Can you work these out from the model? Positions are in its coordinate system, mm. A direction names the side the tool comes from. Coordinates: 2 decimals unless noted, no trailing zeros. Order: outer loops, then holes, each group sorted by start corner. A loop starts at its lowest first (then second) coordinate and runs counter-clockwise, first axis right, second up. Notation, with made-up numbers: (36.25, 19.25) -> (56.25, 19.25) arc R10 cw to (56.25, 38.25) -> close; hole circle Ø10 at (-35.75, 37). An arc over 180 degrees is marked (long way). Return JSON: item names as keys, results as strings. Group by question number.
1) For pin 1 (3 mm diameter, centred on y = 23, z = -14.5, fed in from -X); pin 2 (14 mm diameter, centred on x = 27, z = 3.5, fed in from +Y); pin 3 (3 mm diameter, centred on x = 5.5, y = -11, fed in from -Z), each with a flat end and sliding along its axis, tell me the tip position at first contact or that it passes through.
2) For faces 5 (the flat face through (-34, 9, 18)), 6 (the flat face through (0, 0, 24)), 7 (the flat face through (1, 0, 22)), 8 (the cylindrical face through (45.186, 19.524, 7.336)), 9 (the flat face through (33, 25, 8)), which set-ups out of +Z, -Z, +X, -X, +Y, -Y let a thin tool reach every point of the face, with its end or its side?
3) Thinking about a two-plate mould opening in X: for faces 1 (the flat face through (-36.2, 9.1, 20)), 2 (the flat face through (33.4, 11.4, -18)), 3 (the cylindrical face through (-8.02, -36.12, -20.99)), 4 (the flat face through (46.2, -17, 14)), which applies, +X half, -X half, draft (parallel to the pull), parting line (faces both ways), or undercut?
4) If we section it at A-A, the plane y = 0: State how many separate pieces and enclosed holes the cut face has, then the cut area to 3 significant figures.
5) If we section it at C-C, the plane z = 3: Please give me the cut outline in (x, y), then the cut area to 3 significant figures.
6) If we section it at B-B, the plane x = -27: Please give me the cut outline in (y, z), then the cut area to 3 significant figures.
7) If I drill on probe 1 along Z at (x, y) = (33.5, 12); probe 2 along Z at (x, y) = (-19, -29.5); probe 3 along Y at (x, z) = (40, 6), over which ranges is the centre line in solid material (lowest first)? Write a range as from..to.
Autodesk Inventor part; units mm, degrees
ref_plane "作業平面1" through (0, 0, 0) normal (1, 0, 0) x (0, 1, 0)
ref_plane "YZ Plane" through (0, 0, 0) normal (1, 0, 0) x (0, 1, 0)
ref_plane "XZ Plane" through (0, 0, 0) normal (0, 1, 0) x (-1, 0, 0)
sketch "ｽｹｯﾁ1" plane through (0, 0, 0) normal (0, 0, 1) x (1, 0, 0)
  circle A0 centre (0, 0) radius 40
  dimension "d0" = 80
extrude "押し出し1" add sketch "ｽｹｯﾁ1" along normal mid plane 40
sketch "ｽｹｯﾁ2" plane through (0, 0, 20) normal (0, 0, 1) x (1, 0, 0)
  circle A0 centre (0, 0) radius 40
  circle A1 centre (0, 0) radius 37
  dimension "d3" = 3
extrude "押し出し2" add sketch "ｽｹｯﾁ2" along normal blind 2 contours A1
mirror "Mirror1" about plane through (0, 0, 0) normal (0, 0, 1) of "押し出し2"
ref_plane "作業平面1" through (0, 0, 0) normal (1, 0, 0) x (0, 1, 0)
sketch "ｽｹｯﾁ3" plane through (0, 0, 0) normal (1, 0, 0) x (0, 1, 0)
  line L0 (-37, -22) -> (37, -22)
  line L1 (40, -20) -> (-40, -20)
  line L2 (-25, 26) -> (25, 26)
  line L3 (25, 26) -> (25, -20)
  line L4 (25, -20) -> (-25, -20)
  line L5 (-25, -20) -> (-25, 26)
  line L6 (-25, 3) -> (25, 3)
  line L7 (0, 26) -> (0, -20)
  line L8 (0, -20) -> (0, 24.715)
  dimension "d6" = 50
  dimension "d7" = 46
  dimension "d8" = 25
extrude "押し出し3" add sketch "ｽｹｯﾁ3" along normal blind 46.2
sketch "Sketch4" plane through (46.2, 0, 0) normal (1, 0, 0) x (0, 0, -1)
  point P0 (0, 0)
ref_plane "Work Plane2" through (46.2, 0, -20) normal (0, -1, 0) x (1, 0, 0)
ref_plane "Work Plane3" through (46.2, 25, 3) normal (0, 0, -1) x (-1, 0, 0)
shell "Shell1" thickness 2 removed faces 0
sketch "Sketch7" plane through (0, 0, 22) normal (0, 0, 1) x (1, 0, 0)
  circle A0 centre (0, 0) radius 37
hole "Hole1" at (0, 0, 22) direction (0, 0, -1) diameter 50 end through all
sketch "Sketch8" plane through (46.2, 0, 0) normal (1, 0, 0) x (0, 0, -1)
  point P0 (-3, 0)
hole "Hole2" at (46.2, 0, 3) direction (-1, 0, 0) diameter 40 depth 2 tip angle 118
sketch "Sketch9" plane through (0, 0, -22) normal (0, 0, -1) x (-1, 0, 0)
  circle A0 centre (0, 0) radius 25
extrude "Extrusion7" add sketch "Sketch9" against normal blind 10
sketch "Sketch10" plane through (0, 0, -22) normal (0, 0, -1) x (-1, 0, 0)
  circle A0 centre (0, 0) radius 25
  circle A1 centre (0, 0) radius 25
extrude "Extrusion8" cut sketch "Sketch10" against normal blind 10
properties part number "Robot-Axis5"
Result sheet:
{
 "1": {"pin 1": "stops at x = -33.73", "pin 2": "stops at y = 34.64", "pin 3": "stops at z = 24"},
 "2": {"face 5": "none", "face 6": "+Z, -Z, -X, +Y, -Y", "face 7": "-Z", "face 8": "+X", "face 9": "+Z, +X, +Y"},
 "3": {"face 1": "draft", "face 2": "undercut", "face 3": "parting line", "face 4": "+X half"},
 "4": {"separate pieces": "3", "enclosed holes": "0", "area": "287 mm2"},
 "5": {"outline": "(30.25, -23) arc R38 cw (long way) to (30.25, 23) -> (44.2, 23) -> (44.2, 20) -> (46.2, 20) -> (46.2, 25) -> (31.22, 25) arc R40 ccw (long way) to (31.22, -25) -> (46.2, -25) -> (46.2, -20) -> (44.2, -20) -> (44.2, -23) -> close", "area": "461 mm2"},
 "6": {"outline": "(-29.51, -20) -> (-25.3, -20) -> (-25.3, -22) -> (25.3, -22) -> (25.3, -20) -> (29.51, -20) -> (29.51, 20) -> (25.3, 20) -> (25.3, 22) -> (-25.3, 22) -> (-25.3, 20) -> (-29.51, 20) -> close; hole (-26.74, -18) -> (-22.27, -18) -> (-22.27, -20) -> (22.27, -20) -> (22.27, -18) -> (26.74, -18) -> (26.74, 18) -> (22.27, 18) -> (22.27, 20) -> (-22.27, 20) -> (-22.27, 18) -> (-26.74, 18) -> close", "area": "460 mm2"},
 "7": {"probe 1": "z = -22..-18, 24..26", "probe 2": "z = -22..-18, 18..22", "probe 3": "y = -25..-23, 23..25"}
}
